```python
from build123d import *

# Parameters (mm, degrees)
SKETCH1_W           = 30
SKETCH1_H           = 25
SKETCH1_R           = 1.45
BOSS_EXTRUDE1_DEPTH = 18
SKETCH3_W           = 30
SKETCH3_H           = 25
BOSS_EXTRUDE2_DEPTH = 2
SKETCH4_W           = 24
SKETCH4_H           = 16
CUT_EXTRUDE2_DEPTH  = 26
SKETCH5_W           = 25
SKETCH5_H           = 2
BOSS_EXTRUDE3_DEPTH = 10
BOSS_EXTRUDE4_DEPTH = 2
BOSS_EXTRUDE5_DEPTH = 10


with BuildPart() as part:
    # Sketch1 → Boss-Extrude1 (new body)
    with BuildSketch(Plane(origin=(0, 0, 0), x_dir=(1, 0, 0), z_dir=(0, 1, 0))):
        with Locations((4.678899083, -0.940366972)):
            Rectangle(SKETCH1_W, SKETCH1_H)
        with Locations((-3.071100917, 7.559633028)):
            Circle(SKETCH1_R, mode=Mode.SUBTRACT)
        with Locations((12.428899083, 7.559633028)):
            Circle(SKETCH1_R, mode=Mode.SUBTRACT)
        with Locations((12.428899083, -9.440366972)):
            Circle(SKETCH1_R, mode=Mode.SUBTRACT)
        with Locations((-3.071100917, -9.440366972)):
            Circle(SKETCH1_R, mode=Mode.SUBTRACT)
    extrude(amount=BOSS_EXTRUDE1_DEPTH)

    # Sketch3 → Boss-Extrude2 (add)
    with BuildSketch(Plane(origin=(0, 18, 0), x_dir=(1, 0, 0), z_dir=(0, 1, 0))):
        with Locations((4.678899083, -0.940366972)):
            Rectangle(SKETCH3_W, SKETCH3_H)
    extrude(amount=BOSS_EXTRUDE2_DEPTH)

    # Sketch4 → Cut-Extrude2 (cut, through all)
    with BuildSketch(Plane.XY.offset(13.440366972)):
        with Locations((4.678899083, 10)):
            Rectangle(SKETCH4_W, SKETCH4_H)
    extrude(amount=-CUT_EXTRUDE2_DEPTH, mode=Mode.SUBTRACT)

    # Sketch5 → Boss-Extrude3 (add)
    with BuildSketch(Plane(origin=(19.678899083, 0, 0), x_dir=(0, 0, -1), z_dir=(1, 0, 0))):
        with Locations((-0.940366972, 19)):
            Rectangle(SKETCH5_W, SKETCH5_H)
    extrude(amount=BOSS_EXTRUDE3_DEPTH)

    # Sketch6 → Boss-Extrude4 (add)
    with BuildSketch(Plane(origin=(0, 20, 0), x_dir=(1, 0, 0), z_dir=(0, 1, 0))):
        Polygon((19.678899083, 11.559633028), (19.678899083, 61.559633028), (9.678899083, 61.054804674), (9.678899083, 11.559633028), align=None)
        Polygon((29.678899083, 62.064461381), (19.678899083, 61.559633028), (19.678899083, 11.559633028), (29.678899083, 11.559633028), align=None)
        Polygon((29.678899083, -13.440366972), (19.678899083, -13.440366972), (19.678899083, -63.440366972), (29.678899083, -63.945195326), align=None)
        Polygon((19.678899083, -63.440366972), (19.678899083, -13.440366972), (9.678899083, -13.440366972), (9.678899083, -62.935538619), align=None)
    extrude(amount=-BOSS_EXTRUDE4_DEPTH)

    # Sketch7 → Boss-Extrude5 (add)
    with BuildSketch(Plane(origin=(0, 20, 0), x_dir=(1, 0, 0), z_dir=(0, 1, 0))):
        Polygon((9.678899083, 61.054804674), (29.678899083, 62.064461381), (29.678899083, 58.064461381), (9.678899083, 57.054804674), align=None)
        Polygon((9.678899083, -58.935538619), (29.678899083, -59.945195326), (29.678899083, -63.945195326), (9.678899083, -62.935538619), align=None)
    extrude(amount=BOSS_EXTRUDE5_DEPTH)


solid = part.part
```
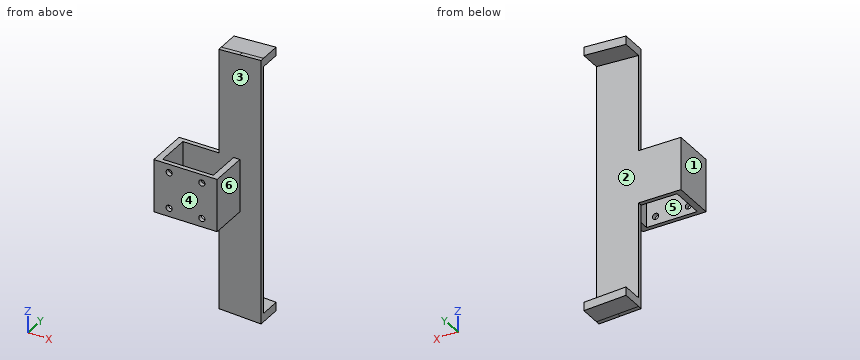
Verification items for the finished model (mm, model axes). Face numbers are marked on the shaded views. A direction names the side the tool comes from. Give positions to 0.01 mm unless a question says otherwise; leave off trailing zeros. Loops run counter-clockwise (first coordinate to the right, second up) from the corner with the lowest first, then second, coordinate; pieces in that order, holes last.
1. Section check C-C, the plane z = -5. Enter the section's corners in (x, y), then the cut area to 3 significant figures.
2. Mould release check, pull along X, two halves, no side actions. Record for the marked faces 1, 2 and 3: released by +X, released by -X, zero draft, split by the parting line, or undercut.
3. Section check A-A, the plane y = 26.5. Enter the section's corners in (x, z).
4. Section check D-D, the plane x = 12.5. Enter the section's corners in (y, z), then the cut area to 3 significant figures.
5. Go/stop test with flat-tipped pins: pin 1 Ø10 at (x, z) = (12, 1) entering from -Y; pin 2 Ø2.5 at (x, z) = (-3.07, -7.56) entering from +Y; pin 3 Ø12 at (y, z) = (9.5, 16) entering from +X; pin 4 Ø10 at (y, z) = (19, -44) entering from -X. Record where each tip stops, or that it passes through.
6. Thickness scan on line 1 (Y direction, x = 0, z = -7.5); line 2 (X direction, y = 18.5, z = 18); line 3 (X direction, y = 12.75, z = -5). Record the ranges inside material, lowest first.
7. Section check B-B, the plane x = 0. Enter the section's corners in (y, z).
8. Set-up check for the marked faces 4, 5 and 6: record each of +Z, -Z, +X, -X, +Y, -Y from which the full face is reachable in a straight line by a thin tool's end or side.
Geometry says:
1. outline: (-10.32, 0) - (19.68, 0) - (19.68, 18) - (29.68, 18) - (29.68, 20) - (-10.32, 20) - close; hole (-7.32, 2) - (16.68, 2) - (16.68, 18) - (-7.32, 18) - close
1. area: 236 mm2
2. face 1: released by -X
2. face 2: zero draft
2. face 3: undercut
3. outline: (9.68, -61.05) - (29.68, -62.06) - (29.68, -58.06) - (9.68, -57.05) - close; (9.68, 58.94) - (29.68, 59.95) - (29.68, 63.95) - (9.68, 62.94) - close
4. outline: (0, -11.56) - (2, -11.56) - (2, -9.01) - (0, -9.01) - close; (0, -6.11) - (2, -6.11) - (2, 7.99) - (0, 7.99) - close; (0, 10.89) - (2, 10.89) - (2, 13.44) - (0, 13.44) - close; (18, -61.2) - (30, -61.2) - (30, -57.2) - (20, -57.2) - (20, 59.08) - (30, 59.08) - (30, 63.08) - (18, 63.08) - close
4. area: 367 mm2
5. pin 1: stops at y = 0
5. pin 2: stops at y = 20
5. pin 3: stops at x = 19.68
5. pin 4: stops at x = 9.68
6. line 1: y = 0 to 2, 18 to 20
6. line 2: x = 9.68 to 29.68
6. line 3: x = -10.32 to -7.32, 16.68 to 19.68
7. outline: (0, -11.56) - (2, -11.56) - (2, 13.44) - (0, 13.44) - close; (18, -11.56) - (20, -11.56) - (20, 13.44) - (18, 13.44) - close
8. face 4: +Z, -Z, +X, -X, -Y
8. face 5: +Z, -Z
8. face 6: +Z, -Z, +X, -Y
